from build123d import *

# Parameters (mm, degrees)
SKETCH1_R           = 1.25
SKETCH1_R_2         = 4
SKETCH1_W           = 2
SKETCH1_H           = 5
BOSS_EXTRUDE1_DEPTH = 5


with BuildPart() as part:
    # Sketch1 → Boss-Extrude1 (new body)
    with BuildSketch(Plane(origin=(0, 0, 0), x_dir=(0, 0, -1), z_dir=(1, 0, 0))):
        with BuildLine():
            Line((-22.5, 0), (-22.5, 90))
            ThreePointArc((-22.5, 90), (0, 102), (22.5, 90))
            Line((22.5, 90), (22.5, 0))
            ThreePointArc((22.5, 0), (0, -12), (-22.5, 0))
        make_face()
        with Locations((0, 7)):
            Circle(SKETCH1_R, mode=Mode.SUBTRACT)
        with Locations((7, 0)):
            Circle(SKETCH1_R, mode=Mode.SUBTRACT)
        with Locations((0, -7)):
            Circle(SKETCH1_R, mode=Mode.SUBTRACT)
        with Locations((-7, 0)):
            Circle(SKETCH1_R, mode=Mode.SUBTRACT)
        with Locations((-10.25, 88.5)):
            Circle(SKETCH1_R, mode=Mode.SUBTRACT)
        with Locations((10.25, 88.5)):
            Circle(SKETCH1_R, mode=Mode.SUBTRACT)
        with Locations((0, 45)):
            Circle(SKETCH1_R_2, mode=Mode.SUBTRACT)
        with Locations((16.5, 73.5)):
            Rectangle(SKETCH1_W, SKETCH1_H, mode=Mode.SUBTRACT)
    extrude(amount=BOSS_EXTRUDE1_DEPTH)


solid = part.part
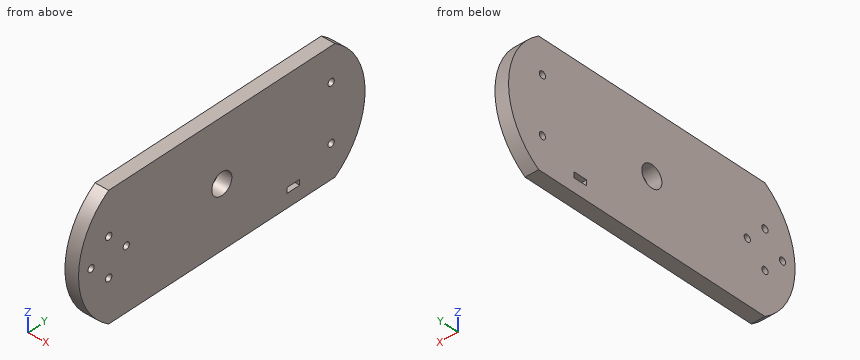
Here's how the part is built. I have some questions about the finished solid (model axes, mm). Coordinates: 2 decimals unless noted, no trailing zeros. Write each loop counter-clockwise with the first axis right and the second up, starting at its lowest first coordinate (ties: lowest second). Pieces come first, ordered by that corner, then holes.
1) If we section it at D-D (z = -7): List the corners of the cut face in (x, y) for me, plus the area to 3 significant figures.
Filled in:
outline: (0, -11.08) - (5, -11.08) - (5, -1.25) - (0, -1.25) - close; (0, 1.25) - (5, 1.25) - (5, 101.08) - (0, 101.08) - close
area: 548 mm2
2) If we section it at A-A (y = 45): List the corners of the cut face in (x, z) for me, plus the area to 3 significant figures.
Filled in:
outline: (0, -22.5) - (5, -22.5) - (5, -4) - (0, -4) - close; (0, 4) - (5, 4) - (5, 22.5) - (0, 22.5) - close
area: 185 mm2
3) If I drill on line 1 (Z direction, x = 3.6, y = 88.5); line 2 (Y direction, x = 2, z = -1); line 3 (Y direction, x = 0.7, z = -10), over which ranges is the centre line in solid material (lowest first)?
Filled in:
line 1: z = -22.5 to -11.5, -9 to 9, 11.5 to 22.5
line 2: y = -11.98 to -7.75, -6.25 to 6.25, 7.75 to 41.13, 48.87 to 101.98
line 3: y = -10.09 to 87.28, 89.72 to 100.09
4) If we section it at B-B (z = 0): List the corners of the cut face in (x, y) for me, plus the area to 3 significant figures.
Filled in:
outline: (0, -12) - (5, -12) - (5, -8.25) - (0, -8.25) - close; (0, -5.75) - (5, -5.75) - (5, 5.75) - (0, 5.75) - close; (0, 8.25) - (5, 8.25) - (5, 41) - (0, 41) - close; (0, 49) - (5, 49) - (5, 102) - (0, 102) - close
area: 505 mm2
5) I'm going to push flat-ended pins straight in: pin 1 (1.5 mm diameter, centred on y = 88.5, z = -10.25, fed in from +X); pin 2 (1 mm diameter, centred on x = 2.5, z = -16.5, fed in from +Y); pin 3 (1 mm diameter, centred on x = 2, z = -17, fed in from -Y). Where does each tip first touch, or does it pass through?
Filled in:
pin 1: passes through
pin 2: stops at y = 96.77
pin 3: stops at y = -6.4
6) If we section it at C-C (x = 1.6): Count the separate pieces of the cut face and the enclosed holes in it, plus the area to 3 significant figures.
Filled in:
separate pieces: 1
enclosed holes: 8
area: 4,720 mm2
